Geometry: final body of the model. Coordinates: model frame, mm. Face numbers are marked on the shaded views. A direction names the side the tool comes from. Give positions to 0.01 mm unless a question says otherwise; leave off trailing zeros. Order: outer loops, then holes, each group sorted by start corner. A loop starts at its lowest first (then second) coordinate and runs counter-clockwise, first axis right, second up. Notation, with made-up numbers: (-1, 81) - (33, 81) arc R18 ccw to (33, 115) - close; hole circle Ø5 at (45, 47.25). An arc over 180 degrees is marked (long way). Write item = value, one per line. Start each with the question number.
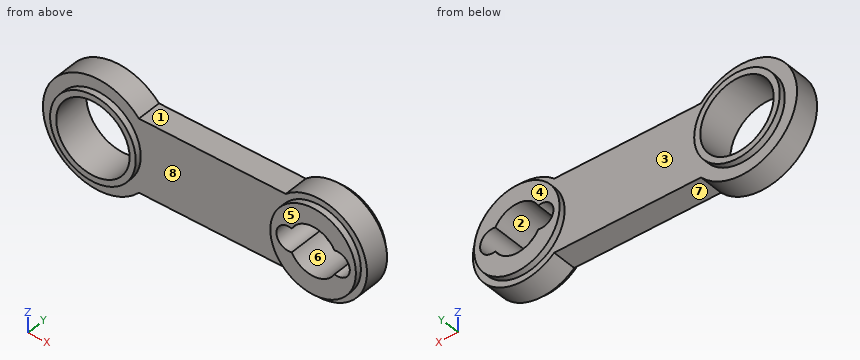
from build123d import *

# Parameters (mm, degrees)
F1_DEPTH = 1
F2_R     = 3.5
F3_DEPTH = 1.5
F4_R     = 3
F5_DEPTH = 3.001


with BuildPart() as f1:
    # F0 (on Front) → F1 (new body, symmetric)
    with BuildSketch(Plane.XZ):
        with BuildLine():
            Line((15.3542486889, 3), (3.3541019662, 3))
            ThreePointArc((3.3541019662, 3), (-4.5, 0), (3.3541019662, -3))
            Line((3.3541019662, -3), (15.3542486889, -3))
            ThreePointArc((15.3542486889, -3), (22, 0), (15.3542486889, 3))
        make_face()
    extrude(amount=F1_DEPTH, both=True)

    # F2 (on Front) → F3 (join, symmetric)
    with BuildSketch(Plane.XZ):
        Circle(F2_R)
        with Locations((18, 0)):
            Circle(F2_R)
    extrude(amount=F3_DEPTH, both=True)

    # F4 (on face) → F5 (cut, through all)
    with BuildSketch(Plane.XZ.offset(1.5)):
        Circle(F4_R)
        with BuildLine():
            ThreePointArc((19.75, -0.9682458366), (21, 0), (19.75, 0.9682458366))
            ThreePointArc((19.75, 0.9682458366), (18, 2), (16.25, 0.9682458366))
            ThreePointArc((16.25, 0.9682458366), (15, 0), (16.25, -0.9682458366))
            ThreePointArc((16.25, -0.9682458366), (18, -2), (19.75, -0.9682458366))
        make_face()
    extrude(amount=-F5_DEPTH, mode=Mode.SUBTRACT)


solid = f1.part
Q1. Material intervals for line 1 along Z through (x, y) = (0, 0.1); line 2 along X through (y, z) = (1.35, 0.5); line 3 along X through (y, z) = (-0.2, 1.5), sorted ascending. Write a range as from..to.
Q2. Pull-direction query (Z, two-part tool) for the marked faces 1, 2 and 3; classes: +Z half, -Z half, draft (parallel to the pull), parting line (faces both ways), or undercut.
Q3. Section D-D, the plane z = 2.75. Return the cut outline in (x, y).
Q4. Set-up query: the marked faces 4, 5, 6, 7 and 8. Return all of +Z, -Z, +X, -X, +Y, -Y with unobstructed straight access to the full face (end or side cutting, diameter ignored); none if empty.
Q5. Contact query for flat-ended pins moving along their axis: pin 1 (3 mm diameter, centred on x = 11.5, z = 1, fed in from -Y); pin 2 (1 mm diameter, centred on x = 10, y = -0.5, fed in from -Z); pin 3 (1.6 mm diameter, centred on x = 9, y = 0.5, fed in from +Z). Output: stop coordinate, or through.
Q6. Section C-C, the plane z = 0. Return the cut outline in (x, y).
Q7. Section A-A, the plane x = 0. Return the cut outline in (y, z), then the cut area to 3 significant figures.
Q8. Section B-B, the plane y = 0.6. Return the cut outline in (x, z), then the cut area to 3 significant figures.
The answers:
q1.line_1 = -4.5..-3, 3..4.5
q1.line_2 = -3.46..-2.96, 2.96..3.46, 14.54..15.13, 20.87..21.46
q1.line_3 = -4.24..-2.6, 2.6..16.68, 19.32..21.71
q2.face_1 = +Z half
q2.face_2 = undercut
q2.face_3 = draft
q3.outline = (-3.56, -1) - (-2.17, -1) - (-2.17, -1.5) - (-1.2, -1.5) - (-1.2, 1.5) - (-2.17, 1.5) - (-2.17, 1) - (-3.56, 1) - close; (1.2, -1.5) - (2.17, -1.5) - (2.17, -1) - (15.83, -1) - (15.83, -1.5) - (20.17, -1.5) - (20.17, -1) - (20.9, -1) - (20.9, 1) - (20.17, 1) - (20.17, 1.5) - (15.83, 1.5) - (15.83, 1) - (2.17, 1) - (2.17, 1.5) - (1.2, 1.5) - close
q4.face_4 = +Z, -Z, +X, -X, +Y
q4.face_5 = +Z, -Z, +X, -X, -Y
q4.face_6 = +Y, -Y
q4.face_7 = -Z, +Y, -Y
q4.face_8 = -Y
q5.pin_1 = -1
q5.pin_2 = -3
q5.pin_3 = 3
q6.outline = (-4.5, -1) - (-3.5, -1) - (-3.5, -1.5) - (-3, -1.5) - (-3, 1.5) - (-3.5, 1.5) - (-3.5, 1) - (-4.5, 1) - close; (3, -1.5) - (3.5, -1.5) - (3.5, -1) - (14.5, -1) - (14.5, -1.5) - (15, -1.5) - (15, 1.5) - (14.5, 1.5) - (14.5, 1) - (3.5, 1) - (3.5, 1.5) - (3, 1.5) - close; (21, -1.5) - (21.5, -1.5) - (21.5, -1) - (22, -1) - (22, 1) - (21.5, 1) - (21.5, 1.5) - (21, 1.5) - close
q7.outline = (-1.5, -3.5) - (-1, -3.5) - (-1, -4.5) - (1, -4.5) - (1, -3.5) - (1.5, -3.5) - (1.5, -3) - (-1.5, -3) - close; (-1.5, 3) - (1.5, 3) - (1.5, 3.5) - (1, 3.5) - (1, 4.5) - (-1, 4.5) - (-1, 3.5) - (-1.5, 3.5) - close
q7.area = 7.00 mm²
q8.outline = (3.35, -3) - (15.35, -3) arc R4 ccw (long way) to (15.35, 3) - (3.35, 3) arc R4.5 ccw (long way) to start; hole circle Ø6 at (0, 0); hole (16.25, -0.97) arc R2 ccw to (19.75, -0.97) arc R1 ccw (long way) to (19.75, 0.97) arc R2 ccw to (16.25, 0.97) arc R1 ccw (long way) to start
q8.area = 131 mm²
